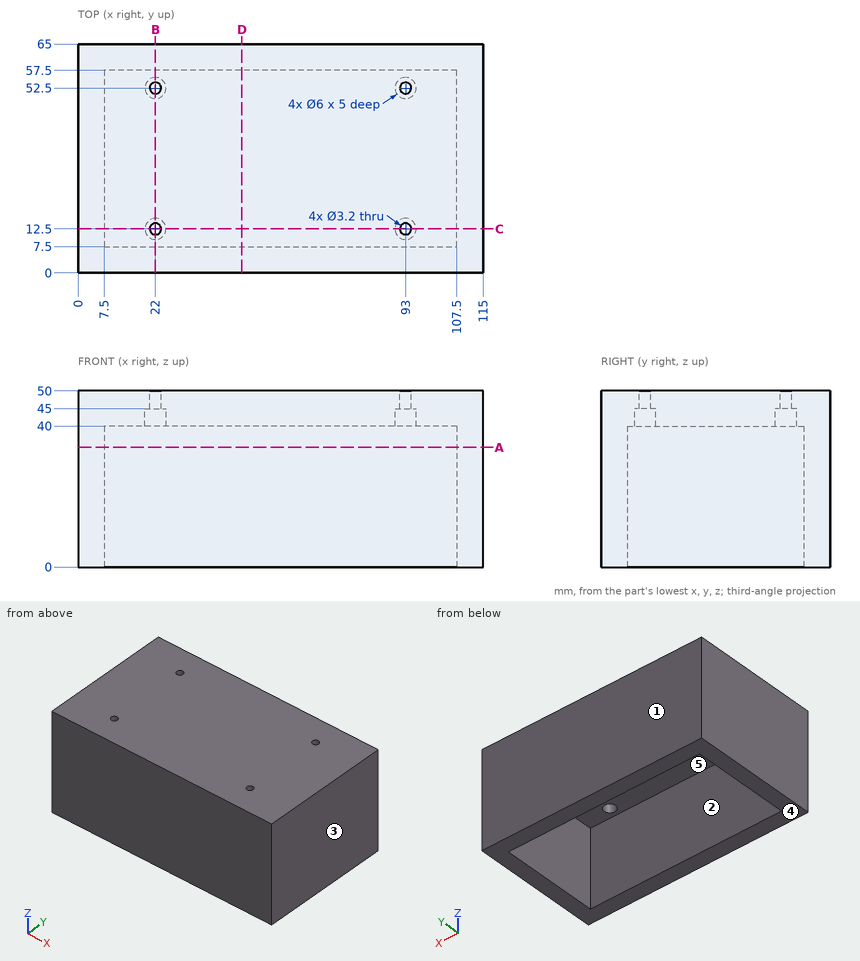
Here's the drawing with two shaded views (mm, measured from the low corner). I have some questions. A direction names the side the tool comes from. Give positions to 0.01 mm unless a question says otherwise; leave off trailing zeros. Order: outer loops, then holes, each group sorted by start corner. A loop starts at its lowest first (then second) coordinate and runs counter-clockwise, first axis right, second up. Notation, with made-up numbers: (12.5, -5.75) - (22.5, -5.75) arc R24 cw to (22.5, 30.25) - close; hole circle Ø1 at (51.25, 57.5). An arc over 180 degrees is marked (long way). Write each question's results on one line, items separated by ' | '.
1) If we mould it in two halves opening along Y, with no side actions, what happens to the marked faces 1, 2 and 3? For each: pulls with the +Y half, pulls with the -Y half, needs draft (parallel to the pull), parting line crosses it, or undercut.
Final values:
face 1: pulls with the +Y half | face 2: undercut | face 3: needs draft
2) Please list where these lines run through material, in increasing order: line 1 along X through (y, z) = (52.5, 42.3); line 2 along Y through (x, z) = (22, 48); line 3 along Y through (x, z) = (22, 42). Write a range as [from, to].
Final values:
line 1: x = [0, 19], [25, 90], [96, 115] | line 2: y = [0, 10.9], [14.1, 50.9], [54.1, 65] | line 3: y = [0, 9.5], [15.5, 49.5], [55.5, 65]
3) On a 3-axis mill with a long thin cutter (end or side, diameter ignored), from which of +Z, -Z, +X, -X, +Y, -Y can I reach the whole of each face in a straight line? I mean the marked faces 4 and 5. Say none if no direction works.
Final values:
face 4: -Z, +X, -X, +Y, -Y | face 5: -Z
4) Suppose I cut it at B-B, the plane x = 22. Write out the boundary of the cut face in (y, z), then the cut area to 3 significant figures.
Final values:
outline: (0, 0) - (7.5, 0) - (7.5, 40) - (9.5, 40) - (9.5, 45) - (10.9, 45) - (10.9, 50) - (0, 50) - close; (14.1, 45) - (15.5, 45) - (15.5, 40) - (49.5, 40) - (49.5, 45) - (50.9, 45) - (50.9, 50) - (14.1, 50) - close; (54.1, 45) - (55.5, 45) - (55.5, 40) - (57.5, 40) - (57.5, 0) - (65, 0) - (65, 50) - (54.1, 50) - close | area: 1,160 mm^2
5) Suppose I cut it at D-D, the plane x = 46.5. Write out the boundary of the cut face in (y, z), then the cut area to 3 significant figures.
Final values:
outline: (0, 0) - (7.5, 0) - (7.5, 40) - (57.5, 40) - (57.5, 0) - (65, 0) - (65, 50) - (0, 50) - close | area: 1,250 mm^2
6) Suppose I cut it at A-A, the plane z = 34. Write out the boundary of the cut face in (x, y).
Final values:
outline: (0, 0) - (115, 0) - (115, 65) - (0, 65) - close; hole (7.5, 7.5) - (107.5, 7.5) - (107.5, 57.5) - (7.5, 57.5) - close
7) I'm going to push flat-ended pins straight in: pin 1 Ø1.5 at (x, y) = (83.5, 55.5) entering from -Z; pin 2 Ø3 at (x, y) = (93, 12.5) entering from -Z; pin 3 Ø1.8 at (x, y) = (92.5, 11.5) entering from -Z. Where does each tip first touch, or does it pass through?
Final values:
pin 1: stops at z = 40 | pin 2: passes through | pin 3: stops at z = 45
8) Suppose I cut it at C-C, the plane y = 12.5. Write out the boundary of the cut face in (x, z), then the cut area to 3 significant figures.
Final values:
outline: (0, 0) - (7.5, 0) - (7.5, 40) - (19, 40) - (19, 45) - (20.4, 45) - (20.4, 50) - (0, 50) - close; (23.6, 45) - (25, 45) - (25, 40) - (90, 40) - (90, 45) - (91.4, 45) - (91.4, 50) - (23.6, 50) - close; (94.6, 45) - (96, 45) - (96, 40) - (107.5, 40) - (107.5, 0) - (115, 0) - (115, 50) - (94.6, 50) - close | area: 1,660 mm^2
